Source: CAD feature listing. Evaluate the final solid. Frame: model axes, mm. A direction names the side the tool comes from. Give positions to 0.01 mm unless a question says otherwise; leave off trailing zeros. Write each loop counter-clockwise with the first axis right and the second up, starting at its lowest first coordinate (ties: lowest second). Pieces come first, ordered by that corner, then holes. Notation, with made-up numbers: (73, 84) -> (121, 84) arc R28 cw to (121, 112) -> close; hole circle Ø10 at (20.25, 0). An arc over 180 degrees is marked (long way). Write item = value, one per line.
from build123d import *

# Parameters (mm, degrees)
SKETCH1_R               = 25.65
SKETCH1_R_2             = 19.65
SKETCH1_R_3             = 4
SKETCH1_R_4             = 0.95
SKETCH1_W               = 40.16
SKETCH1_H               = 20.39
BOSS_EXTRUDE2_DEPTH     = 3.7
SKETCH5_R               = 19.65
SKETCH5_W               = 40.16
SKETCH5_H               = 20.39
BOSS_EXTRUDE3_DEPTH     = 28.1
CUT_EXTRUDE1_REACH      = 108.468
SKETCH6_W               = 40.16
SKETCH6_H               = 28.1
CUT_EXTRUDE2_REACH      = 114.631
CUT_EXTRUDE2_END_RADIUS = 25.65
SKETCH7_W               = 29.863740461
SKETCH7_H               = 10
SKETCH8_R               = 1.45
CUT_EXTRUDE3_DEPTH      = 15
SKETCH9_R               = 0.95
CUT_EXTRUDE4_DEPTH      = 12
CUT_EXTRUDE5_DEPTH      = 104.481486871
FILLET1_R               = 2


with BuildPart() as part:
    # Sketch1 → Boss-Extrude2 (new body)
    # profile 1 of 6: a face of its own
    with BuildSketch(Plane(origin=(0, 0, 0), x_dir=(1, 0, 0), z_dir=(0, 1, 0))):
        Circle(SKETCH1_R)
        Circle(SKETCH1_R_2, mode=Mode.SUBTRACT)
    # profile 2 of 6: a face of its own
    with BuildSketch(Plane(origin=(0, 0, 0), x_dir=(1, 0, 0), z_dir=(0, 1, 0))):
        Circle(SKETCH1_R_2)
        with Locations(Location((0, 0, 0), (0, 0, 270))):
            Circle(SKETCH1_R_3, mode=Mode.SUBTRACT)
        with Locations(Location((16.6, 0, 0), (0, 0, 270))):
            Circle(SKETCH1_R_4, mode=Mode.SUBTRACT)
        with Locations(Location((0, -16.6, 0), (0, 0, 270))):
            Circle(SKETCH1_R_4, mode=Mode.SUBTRACT)
        with Locations(Location((-16.6, 0, 0), (0, 0, 270))):
            Circle(SKETCH1_R_4, mode=Mode.SUBTRACT)
        with Locations(Location((0, 16.6, 0), (0, 0, 270))):
            Circle(SKETCH1_R_4, mode=Mode.SUBTRACT)
    # profile 3 of 6: a face of its own
    with BuildSketch(Plane(origin=(0, 0, 0), x_dir=(1, 0, 0), z_dir=(0, 1, 0))):
        with BuildLine():
            Line((30.65, 18.695), (86.986875612, 18.695))
            ThreePointArc((86.986875612, 18.695), (78.869462663, 23.847948025), (69.425, 25.65))
            Line((69.425, 25.65), (0, 25.65))
            ThreePointArc((0, 25.65), (18.137288937, 18.137288937), (25.65, 0))
            ThreePointArc((25.65, 0), (18.137288937, -18.137288937), (0, -25.65))
            Line((0, -25.65), (69.425, -25.65))
            ThreePointArc((69.425, -25.65), (78.869462663, -23.847948025), (86.986875612, -18.695))
            Line((86.986875612, -18.695), (30.65, -18.695))
            Line((30.65, -18.695), (30.65, 18.695))
        make_face()
    # profile 4 of 6: a face of its own
    with BuildSketch(Plane(origin=(0, 0, 0), x_dir=(1, 0, 0), z_dir=(0, 1, 0))):
        with BuildLine():
            Line((87.81, -17.886147573), (87.81, 17.886147573))
            ThreePointArc((87.81, 17.886147573), (87.402987293, 18.295203548), (86.986875612, 18.695))
            Line((86.986875612, 18.695), (30.65, 18.695))
            Line((30.65, 18.695), (30.65, -18.695))
            Line((30.65, -18.695), (86.986875612, -18.695))
            ThreePointArc((86.986875612, -18.695), (87.402987293, -18.295203548), (87.81, -17.886147573))
        make_face()
        with Locations((59.23, 0)):
            Rectangle(SKETCH1_W, SKETCH1_H, mode=Mode.SUBTRACT)
    # profile 5 of 6: a face of its own
    with BuildSketch(Plane(origin=(0, 0, 0), x_dir=(1, 0, 0), z_dir=(0, 1, 0))):
        with Locations((59.23, 0)):
            Rectangle(SKETCH1_W, SKETCH1_H)
    # profile 6 of 6: a face of its own
    with BuildSketch(Plane(origin=(0, 0, 0), x_dir=(1, 0, 0), z_dir=(0, 1, 0))):
        with BuildLine():
            ThreePointArc((87.81, -17.886147573), (95.075, 0), (87.81, 17.886147573))
            Line((87.81, 17.886147573), (87.81, -17.886147573))
        make_face()
    extrude(amount=BOSS_EXTRUDE2_DEPTH)

    # Sketch5 → Boss-Extrude3 (add)
    # profile 1 of 4: a face of its own
    with BuildSketch(Plane(origin=(0, 3.7, 0), x_dir=(1, 0, 0), z_dir=(0, 1, 0))):
        with BuildLine():
            ThreePointArc((25.65, 0), (18.137288937, 18.137288937), (0, 25.65))
            ThreePointArc((0, 25.65), (-25.65, 0), (0, -25.65))
            ThreePointArc((0, -25.65), (18.137288937, -18.137288937), (25.65, 0))
        make_face()
        with Locations(Location((0, 0, 0), (0, 0, 270))):
            Circle(SKETCH5_R, mode=Mode.SUBTRACT)
    # profile 2 of 4: a face of its own
    with BuildSketch(Plane(origin=(0, 3.7, 0), x_dir=(1, 0, 0), z_dir=(0, 1, 0))):
        with BuildLine():
            ThreePointArc((87.81, 17.886147573), (87.402987293, 18.295203548), (86.986875612, 18.695))
            Line((86.986875612, 18.695), (30.65, 18.695))
            Line((30.65, 18.695), (30.65, -18.695))
            Line((30.65, -18.695), (86.986875612, -18.695))
            ThreePointArc((86.986875612, -18.695), (87.402987293, -18.295203548), (87.81, -17.886147573))
            Line((87.81, -17.886147573), (87.81, 17.886147573))
        make_face()
        with Locations((59.23, 0)):
            Rectangle(SKETCH5_W, SKETCH5_H, mode=Mode.SUBTRACT)
    # profile 3 of 4: a face of its own
    with BuildSketch(Plane(origin=(0, 3.7, 0), x_dir=(1, 0, 0), z_dir=(0, 1, 0))):
        with BuildLine():
            ThreePointArc((86.986875612, 18.695), (78.869462663, 23.847948025), (69.425, 25.65))
            Line((69.425, 25.65), (0, 25.65))
            ThreePointArc((0, 25.65), (18.137288937, 18.137288937), (25.65, 0))
            ThreePointArc((25.65, 0), (18.137288937, -18.137288937), (0, -25.65))
            Line((0, -25.65), (69.425, -25.65))
            ThreePointArc((69.425, -25.65), (78.869462663, -23.847948025), (86.986875612, -18.695))
            Line((86.986875612, -18.695), (30.65, -18.695))
            Line((30.65, -18.695), (30.65, 18.695))
            Line((30.65, 18.695), (86.986875612, 18.695))
        make_face()
    # profile 4 of 4: a face of its own
    with BuildSketch(Plane(origin=(0, 3.7, 0), x_dir=(1, 0, 0), z_dir=(0, 1, 0))):
        with BuildLine():
            ThreePointArc((87.81, -17.886147573), (95.075, 0), (87.81, 17.886147573))
            Line((87.81, 17.886147573), (87.81, -17.886147573))
        make_face()
    extrude(amount=BOSS_EXTRUDE3_DEPTH)

    # Sketch6 → Cut-Extrude1 (cut, up to next)
    with BuildSketch(Plane.XY.offset(-10.195), mode=Mode.PRIVATE) as cut_extrude1_sk1:
        with Locations((59.23, 17.75)):
            Rectangle(SKETCH6_W, SKETCH6_H)
    cut_extrude1_tool1 = extrude(cut_extrude1_sk1.sketch, amount=-CUT_EXTRUDE1_REACH, mode=Mode.PRIVATE) & part.part
    add(cut_extrude1_tool1.solids().sort_by_distance((59.23, 17.75, -10.195))[0], mode=Mode.SUBTRACT)

    # Cut-Extrude2: up to this cylinder (the profile starts inside it)
    cut_extrude2_end = Plane(origin=(69.425, 8.7, 0), z_dir=(0, -1, 0)) * Cylinder(CUT_EXTRUDE2_END_RADIUS, 281.562, mode=Mode.PRIVATE)
    # Sketch7 → Cut-Extrude2 (cut, up to the surface)
    with BuildSketch(Plane.ZY.offset(-79.31), mode=Mode.PRIVATE) as cut_extrude2_sk1:
        with Locations((-8.736870231, 8.7)):
            Rectangle(SKETCH7_W, SKETCH7_H)
    cut_extrude2_tool1 = extrude(cut_extrude2_sk1.sketch, amount=-CUT_EXTRUDE2_REACH, mode=Mode.PRIVATE) & cut_extrude2_end
    add(cut_extrude2_tool1.solids().sort_by_distance((79.31, 8.7, -8.73687))[0], mode=Mode.SUBTRACT)

    # Sketch8 → Cut-Extrude3 (cut)
    with BuildSketch(Plane(origin=(0, 31.8, 0), x_dir=(1, 0, 0), z_dir=(0, 1, 0))):
        with Locations(Location((22.65, 0, 0), (0, 0, 270))):
            Circle(SKETCH8_R)
        with Locations(Location((0, -22.65, 0), (0, 0, 270))):
            Circle(SKETCH8_R)
        with Locations(Location((-22.65, 0, 0), (0, 0, 270))):
            Circle(SKETCH8_R)
        with Locations(Location((0, 22.65, 0), (0, 0, 270))):
            Circle(SKETCH8_R)
    extrude(amount=-CUT_EXTRUDE3_DEPTH, mode=Mode.SUBTRACT)

    # Sketch9 → Cut-Extrude4 (cut)
    with BuildSketch(Plane(origin=(0, 31.8, 0), x_dir=(1, 0, 0), z_dir=(0, 1, 0))):
        with Locations(Location((34.88, -4.95, 0), (0, 0, 270))):
            Circle(SKETCH9_R)
        with Locations(Location((34.88, 4.95, 0), (0, 0, 90))):
            Circle(SKETCH9_R)
        with Locations(Location((82.756875612, -4.95, 0), (0, 0, 90))):
            Circle(SKETCH9_R)
        with Locations(Location((82.756875612, 4.95, 0), (0, 0, 270))):
            Circle(SKETCH9_R)
    extrude(amount=-CUT_EXTRUDE4_DEPTH, mode=Mode.SUBTRACT)

    # Sketch12 → Cut-Extrude5 (cut, through all)
    with BuildSketch(Plane(origin=(0, 31.8, 0), x_dir=(1, 0, 0), z_dir=(0, 1, 0))):
        with BuildLine():
            Line((0, 25.65), (69.425, 25.65))
            ThreePointArc((69.425, 25.65), (78.19711491, 24.103371134), (85.911357997, 19.65))
            Line((85.911357997, 19.65), (16.486357997, 19.65))
            ThreePointArc((16.486357997, 19.65), (8.77211491, 24.103371134), (0, 25.65))
        make_face()
        with BuildLine():
            Line((0, -25.65), (69.425, -25.65))
            ThreePointArc((69.425, -25.65), (78.19711491, -24.103371134), (85.911357997, -19.65))
            Line((85.911357997, -19.65), (16.486357997, -19.65))
            ThreePointArc((16.486357997, -19.65), (8.77211491, -24.103371134), (0, -25.65))
        make_face()
    extrude(amount=-CUT_EXTRUDE5_DEPTH, mode=Mode.SUBTRACT)

    # Fillet1
    fillet1_edges = [part.edges().sort_by_distance(p)[0] for p in [
        (39.15, 17.75, -19.65),
        (79.31, 22.75, -19.65),
    ]]
    fillet(fillet1_edges, radius=FILLET1_R)


solid = part.part
(1) Section query D-D (x = 73). Return loops of the section in (y, z) (3 decimals).
Values follow:
outline = (0, -19.65) -> (3.7, -19.65) -> (3.7, 10.195) -> (31.8, 10.195) -> (31.8, 19.65) -> (0, 19.65) -> close
(2) Section query C-C (z = 14). Return loops of the section in (x, y).
Values follow:
outline = (-21.49, 0) -> (90.92, 0) -> (90.92, 31.8) -> (13.79, 31.8) -> (13.79, 3.7) -> (-13.79, 3.7) -> (-13.79, 31.8) -> (-21.49, 31.8) -> close
(3) Section query A-A (x = 22.65). Return loops of the section in (y, z).
Values follow:
outline = (0, -19.65) -> (31.8, -19.65) -> (31.8, -1.45) -> (16.8, -1.45) -> (16.8, 1.45) -> (31.8, 1.45) -> (31.8, 19.65) -> (0, 19.65) -> close
(4) Section query B-B (y = 29). Give the number of separate pieces and of enclosed holes in the cut face, plus the area to 3 significant figures.
Values follow:
separate_pieces = 1
enclosed_holes = 9
area = 2,340 mm2
(5) Access query for faces 1 (the face through (87, 13.7, -7)), 2 (the face through (36, 13, -19.65)), 3 (the face through (39.15, 18, -4)), 4 (the face through (34, 0, 0)), 5 (the face through (0, 3.7, -5)). Directions: +Z, -Z, +X, -X, +Y, -Y. A direction counts if a zero-diameter tool reaches every point of the face in a straight line with its end or side. Return the directions, or none.
Values follow:
face_1 = -Z, +X
face_2 = -Z, +X, +Y, -Y
face_3 = -Z, +Y
face_4 = +Z, -Z, +X, -X, -Y
face_5 = +Y
(6) Material intervals for line 1 (X direction, y = 25, z = 0) (3 decimals); line 2 (Y direction, x = 79.5, z = -8); line 3 (X direction, y = 21, z = 3.5), sorted ascending.
Values follow:
line_1 = -25.65 to -24.1, -21.2 to -19.65, 19.65 to 21.2, 24.1 to 39.15, 79.31 to 95.075
line_2 = 0 to 3.7, 13.7 to 31.8
line_3 = -25.41 to -19.34, 19.34 to 39.15, 79.31 to 94.84
(7) First-contact query: pin 1 (3 mm diameter, centred on y = 28.5, z = -6.5, fed in from +X); pin 2 (1 mm diameter, centred on x = 23, y = 27.5, fed in from +Z); pin 3 (3 mm diameter, centred on x = -16.6, z = 0, fed in from +Y). Flat tips, straight axial feed; report the tip coordinate or a pass-through.
Values follow:
pin_1 = 94.58
pin_2 = 19.65
pin_3 = 3.7
(8) Pull-direction query (Z, two-part tool) for faces 6 (the face through (52, 16, 19.65)), 7 (the face through (34, 31.8, 0)), 8 (the face through (-3.905, 1.824, -0.867)); classes: pulls with the +Z half, pulls with the -Z half, needs draft (parallel to the pull), parting line crosses it, or undercut.
Values follow:
face_6 = pulls with the +Z half
face_7 = needs draft
face_8 = undercut
